Check sheet for the drawn part. Datum: minimum x, y, z corner. Units: mm. A direction names the side the tool comes from. Give positions to 0.01 mm unless a question says otherwise; leave off trailing zeros. Write each loop counter-clockwise with the first axis right and the second up, starting at its lowest first coordinate (ties: lowest second). Pieces come first, ordered by that corner, then holes. Notation, with made-up numbers: (23.25, -9.5) - (36.25, -9.5) arc R27 cw to (36.25, 15.5) - close; hole circle Ø4 at (85, -13.5). An arc over 180 degrees is marked (long way). One line per question, with ' | ' between items. Start each with the question number.
Q1. Thickness scan on L1, parallel to Y at x = 35, z = 4.5; L2, parallel to Y at x = 12.5, z = 48; L3, parallel to Y at x = 24, z = 49.5. Record the ranges inside material, lowest first. Write a range as [from, to].
Q2. Section check D-D on x = 35.5. Record the boundary of the cut face in (y, z).
Q3. Section check A-A on x = 24. Record the boundary of the cut face in (y, z).
Q4. Set-up check for the marked faces 5, 6 and 7: record each of +Z, -Z, +X, -X, +Y, -Y from which the full face is reachable in a straight line by a thin tool's end or side.
Q5. Section check B-B on z = 10. Record the boundary of the cut face in (x, y).
Q6. Release check for a two-part mould opening along X. For the marked faces 1, 2, 3 and 4 record: +X half, -X half, draft (parallel to the pull), parting line (faces both ways), or undercut.
Q7. Section check C-C on y = 32. Record the boundary of the cut face in (x, z), and give its area (3 significant figures).
Q8. Gauge pin test, flat ends, axial feed: P1, Ø3, axis at y = 54, z = 46, coming from the -X side; P2, Ø2, axis at x = 43, z = 53, coming from the -Y side; P3, Ø3.5, axis at x = 44, z = 18, coming from the +Y side; P4, Ø12, axis at x = 25, y = 21, coming from the +Z side (1 decimal). Record the tip position at first contact, or that the pin passes through.
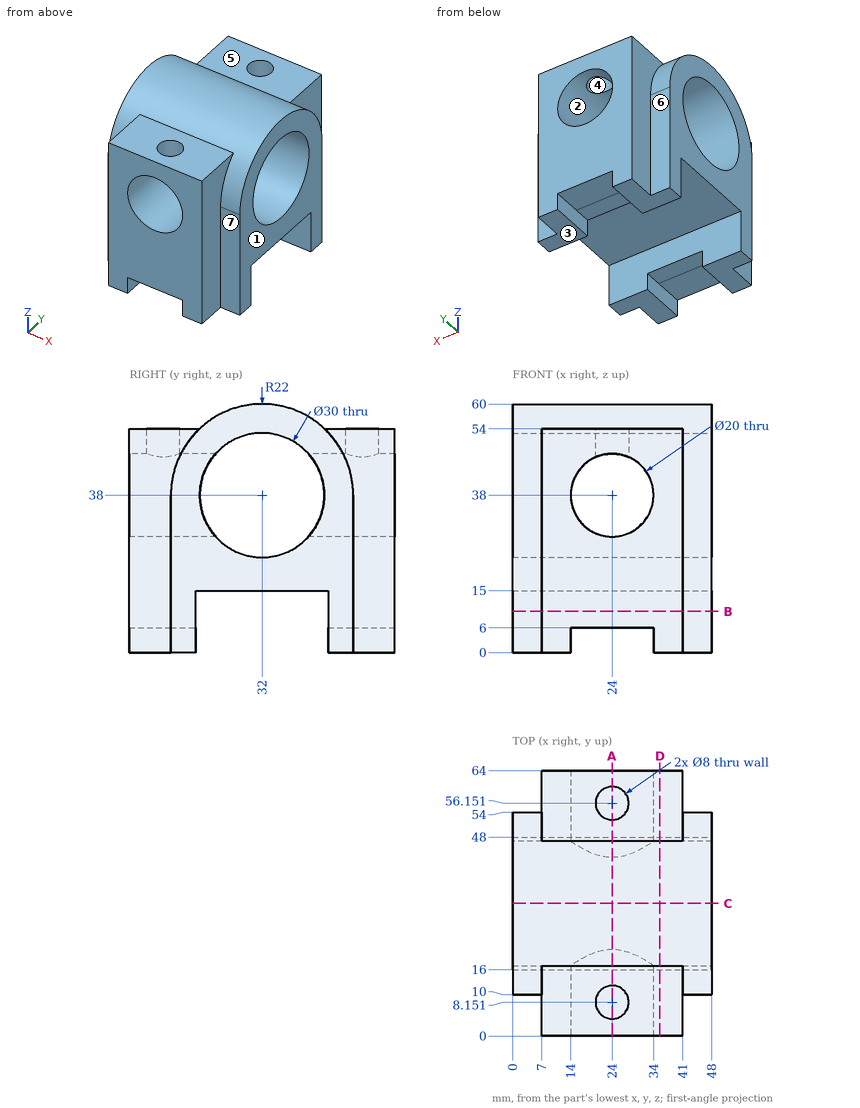
Working result:
1) L1: y = [0, 16], [48, 64] | L2: y = [0, 20.82], [43.18, 64] | L3: y = [0, 4.15], [12.15, 22.37], [41.63, 52.15], [60.15, 64]
2) outline: (0, 0) - (16, 0) - (16, 15) - (48, 15) - (48, 0) - (64, 0) - (64, 54) - (47.1, 54) arc R22 ccw to (16.9, 54) - (0, 54) - close; hole circle Ø30 at (32, 38)
3) outline: (0, 6) - (16, 6) - (16, 15) - (48, 15) - (48, 6) - (64, 6) - (64, 28) - (43.18, 28) arc R15 cw to (20.82, 28) - (0, 28) - close; (0, 48) - (4.15, 48) - (4.15, 54) - (0, 54) - close; (12.15, 48) - (20.82, 48) arc R15 cw to (43.18, 48) - (52.15, 48) - (52.15, 54) - (47.1, 54) arc R22 ccw to (16.9, 54) - (12.15, 54) - close; (60.15, 48) - (64, 48) - (64, 54) - (60.15, 54) - close
4) face 5: +Z, +X, -X, +Y | face 6: +Z, -Z, -X, +Y | face 7: +Z, -Z, +X, -Y
5) outline: (0, 10) - (7, 10) - (7, 0) - (41, 0) - (41, 10) - (48, 10) - (48, 16) - (0, 16) - close; (0, 48) - (48, 48) - (48, 54) - (41, 54) - (41, 64) - (7, 64) - (7, 54) - (0, 54) - close
6) face 1: +X half | face 2: undercut | face 3: draft | face 4: undercut
7) outline: (0, 15) - (48, 15) - (48, 23) - (0, 23) - close; (0, 53) - (48, 53) - (48, 60) - (0, 60) - close | area: 720 mm2
8) P1: stops at x = 0 | P2: stops at y = 15.03 | P3: stops at y = 54 | P4: stops at z = 59.4
